Read the model definition and answer for the solid it produces. Units are mm, in the model's axes. Coordinates: 2 decimals unless noted, no trailing zeros. Loops run counter-clockwise (first coordinate to the right, second up) from the corner with the lowest first, then second, coordinate; pieces in that order, holes last.
from build123d import *

# Parameters (mm, degrees)
SKIZZE1_W                        = 121
SKIZZE1_H                        = 83
AUFSATZ_LINEAR_AUSTRAGEN1_DEPTH  = 1.2
SKIZZE2_R                        = 0.75
SKIZZE2_W                        = 14
SKIZZE2_H                        = 8.25
SKIZZE2_W_2                      = 2.55
SKIZZE2_H_2                      = 2.71
SKIZZE2_W_3                      = 6.6
SKIZZE2_H_3                      = 12
SKIZZE2_W_4                      = 7.6
SKIZZE2_H_4                      = 3.09
SKIZZE2_W_5                      = 2.6
SKIZZE2_H_5                      = 2.314480995
SCHNITT_LINEAR_AUSTRAGEN1_DEPTH  = 105.747028597
F_0_5_0_5_DURCHMESSER_BOHRUNG1_D = 0.5
VERRUNDUNG1_R                    = 3
SCHNITT_LINEAR_AUSTRAGEN2_DEPTH  = 105.747028597
SKIZZE8_W                        = 3.801252581
SKIZZE8_H                        = 8
SKIZZE8_W_2                      = 2.67743865
SCHNITT_LINEAR_AUSTRAGEN3_DEPTH  = 105.747028597
VERRUNDUNG2_R                    = 0.5


with BuildPart() as part:
    # Skizze1 → Aufsatz-Linear austragen1 (new body)
    with BuildSketch(Plane.XY):
        with Locations((0, 44)):
            Rectangle(SKIZZE1_W, SKIZZE1_H)
    extrude(amount=AUFSATZ_LINEAR_AUSTRAGEN1_DEPTH)

    # Skizze2 → Schnitt-Linear austragen1 (cut, through all)
    with BuildSketch(Plane.XY):
        with Locations((42, 61)):
            Circle(SKIZZE2_R)
        with Locations((0, 57.8)):
            Circle(SKIZZE2_R)
        with Locations((0, 23)):
            Circle(SKIZZE2_R)
        with Locations((39.4, 33.8)):
            Circle(SKIZZE2_R)
        with Locations((-26.3, 16.2)):
            Circle(SKIZZE2_R)
        with Locations((-36.389998649, 82.246892958)):
            Circle(SKIZZE2_R)
        with Locations((-49.909999351, 82.246892958)):
            Circle(SKIZZE2_R)
        with Locations((-56.333799461, 20.907941573)):
            Circle(SKIZZE2_R)
        with Locations((53.283097528, 20.907941573)):
            Circle(SKIZZE2_R)
        with Locations((28.5, 6.625)):
            Rectangle(SKIZZE2_W, SKIZZE2_H)
        with Locations((-51, 41)):
            Rectangle(SKIZZE2_W_2, SKIZZE2_H_2)
        with Locations((51, 41)):
            Rectangle(SKIZZE2_W_2, SKIZZE2_H_2)
        with Locations((48.5, 8.5)):
            Rectangle(SKIZZE2_W_3, SKIZZE2_H_3)
        with Locations((-29, 78.5)):
            Rectangle(SKIZZE2_W_4, SKIZZE2_H_4)
        with Locations((20.261326432, 23.962336547)):
            Rectangle(SKIZZE2_W_5, SKIZZE2_H_5)
    extrude(amount=SCHNITT_LINEAR_AUSTRAGEN1_DEPTH, mode=Mode.SUBTRACT)

    # Ø0.5 (0.5) Durchmesser Bohrung1 (through all)
    with Locations(Plane(origin=(0, 0, 0), x_dir=(1, 0, 0), z_dir=(0, 0, -1))):
        with Locations((58.1, -83.1), (38, -83.1), (0, -83.1), (-58.1, -83.1), (-58.1, -59.1), (-58.1, -41.1), (-36.3, -42.1), (-58.1, -4.9), (-36, -4.9), (-14, -4.9), (14, -4.9), (58.1, -4.9), (39.8, -11.3), (58.1, -40.9), (58.1, -22.9), (23.5, -43.8), (18.5, -17.3)):
            Hole(F_0_5_0_5_DURCHMESSER_BOHRUNG1_D / 2)

    # Verrundung1
    verrundung1_edges = [part.edges().sort_by_distance(p)[0] for p in [
        (-60.5, 2.5, 0.6),
        (-60.5, 85.5, 0.6),
        (60.5, 85.5, 0.6),
        (60.5, 2.5, 0.6),
    ]]
    fillet(verrundung1_edges, radius=VERRUNDUNG1_R)

    # Skizze7 → Schnitt-Linear austragen2 (cut, through all)
    with BuildSketch(Plane.XY):
        with BuildLine():
            Line((19.55, 85), (19.55, 87.452976337))
            ThreePointArc((19.55, 87.452976337), (20.5, 88.402976337), (21.45, 87.452976337))
            Line((21.45, 87.452976337), (21.45, 85))
            ThreePointArc((21.45, 85), (20.5, 84.05), (19.55, 85))
        make_face()
        with BuildLine():
            Line((-21.45, 85), (-21.45, 88.302996714))
            ThreePointArc((-21.45, 88.302996714), (-20.5, 89.252996714), (-19.55, 88.302996714))
            Line((-19.55, 88.302996714), (-19.55, 85))
            ThreePointArc((-19.55, 85), (-20.5, 84.05), (-21.45, 85))
        make_face()
        with BuildLine():
            Line((41.95, 3.7), (41.95, -5.660796072))
            ThreePointArc((41.95, -5.660796072), (41, -6.610796072), (40.05, -5.660796072))
            Line((40.05, -5.660796072), (40.05, 3.7))
            ThreePointArc((40.05, 3.7), (41, 4.65), (41.95, 3.7))
        make_face()
        with BuildLine():
            Line((0.95, 3.7), (0.95, -1.929493841))
            ThreePointArc((0.95, -1.929493841), (0, -2.879493841), (-0.95, -1.929493841))
            Line((-0.95, -1.929493841), (-0.95, 3.7))
            ThreePointArc((-0.95, 3.7), (0, 4.65), (0.95, 3.7))
        make_face()
        with BuildLine():
            Line((-46.05, 3.7), (-46.05, -0.870122008))
            ThreePointArc((-46.05, -0.870122008), (-47, -1.820122008), (-47.95, -0.870122008))
            Line((-47.95, -0.870122008), (-47.95, 3.7))
            ThreePointArc((-47.95, 3.7), (-47, 4.65), (-46.05, 3.7))
        make_face()
    extrude(amount=SCHNITT_LINEAR_AUSTRAGEN2_DEPTH, mode=Mode.SUBTRACT)

    # Skizze8 → Schnitt-Linear austragen3 (cut, through all)
    with BuildSketch(Plane.XY):
        with Locations((-60.900626291, 67)):
            Rectangle(SKIZZE8_W, SKIZZE8_H)
        with Locations((60.338719325, 67)):
            Rectangle(SKIZZE8_W_2, SKIZZE8_H)
    extrude(amount=SCHNITT_LINEAR_AUSTRAGEN3_DEPTH, mode=Mode.SUBTRACT)

    # Verrundung2
    verrundung2_edges = [part.edges().sort_by_distance(p)[0] for p in [
        (-59, 71, 0.6),
        (-59, 63, 0.6),
        (59, 63, 0.6),
        (59, 71, 0.6),
    ]]
    fillet(verrundung2_edges, radius=VERRUNDUNG2_R)


solid = part.part
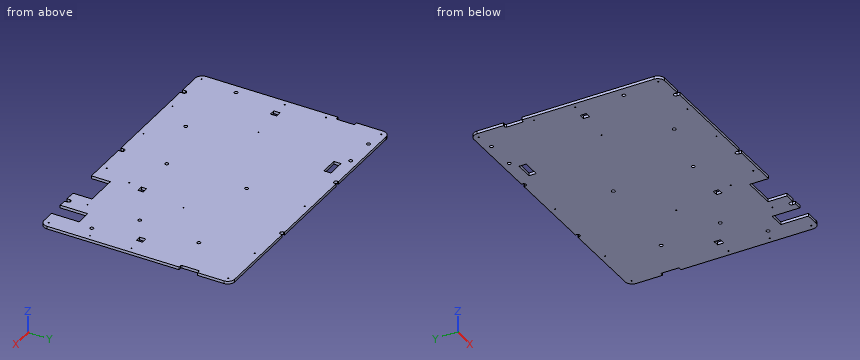
Q1. A cutting plane is placed at C-C (z = 0.45). Count the separate pieces of the cut face and the enclosed holes in it, then the cut area to 3 significant figures.
Findings below:
separate pieces: 1
enclosed holes: 30
area: 9,740 mm2
Q2. Flat-ended cylindrical pins translate along their axes: pin 1 Ø0.6 at (y, z) = (3, 1) entering from -X; pin 2 Ø0.9 at (x, y) = (-26.3, 16.2) entering from +Z; pin 3 Ø0.6 at (y, z) = (85.5, 0.5) entering from +X; pin 4 Ø0.6 at (y, z) = (3.5, 0.5) entering from +X. Find the tip coordinate at first contact, or state that the pin passes through.
Findings below:
pin 1: stops at x = -59.54
pin 2: passes through
pin 3: stops at x = 58.81
pin 4: stops at x = 59.97
Q3. Straight lines are drawn through the part: probe 1 along X at (y, z) = (22.9, 0.5); probe 2 along X at (y, z) = (17.3, 0.75); probe 3 along Y at (x, z) = (39.5, 0.65). For each, find the intervals that lie inside material, in ascending order.
Findings below:
probe 1: x = -60.5 to -0.74, 0.74 to 18.96, 21.56 to 57.85, 58.35 to 60.5
probe 2: x = -60.5 to 18.25, 18.75 to 60.5
probe 3: y = 2.5 to 33.06, 34.54 to 85.5
Q4. A cutting plane is placed at B-B (x = 27.5). Give the vertices of the cut face in (y, z).
Findings below:
outline: (10.75, 0) - (85.5, 0) - (85.5, 1.2) - (10.75, 1.2) - close
Q5. A cutting plane is placed at A-A (y = 69). Give the vertices of the cut face in (x, z).
Findings below:
outline: (-59, 0) - (59, 0) - (59, 1.2) - (-59, 1.2) - close
